Model file for the job. Use its own axes, mm. Face numbers are marked on the shaded views. Round coordinates to 2 decimals unless told otherwise and drop trailing zeros. Write each loop counter-clockwise with the first axis right and the second up, starting at its lowest first coordinate (ties: lowest second). Pieces come first, ordered by that corner, then holes.
```python
from build123d import *

# Parameters (mm, degrees)
F0_R     = 53.4294983316
F0_R_2   = 51.6
F1_DEPTH = 3
F3_R     = 53.9566734819
F4_DEPTH = 2
F5_R     = 1.99999
F6_R     = 37.4035262833
F7_DEPTH = 3
F8_SIZE2 = 1
F8_SIZE  = 1


# Not quite as in the source:
# - a fillet or chamfer is up to 0.001 mm smaller than in the source, because OpenCascade refuses the exact size


with BuildPart() as f1:
    # F0 (on Top) → F1 (new body)
    with BuildSketch(Plane.XY):
        Circle(F0_R)
        Circle(F0_R_2, mode=Mode.SUBTRACT)
    extrude(amount=-F1_DEPTH)

    # F3 (on offset) → F4 (join)
    with BuildSketch(Plane.XY):
        Circle(F3_R)
    extrude(amount=F4_DEPTH)

    # F5 (radius 2 in the source; OpenCascade refuses exactly that, so slightly less here)
    f5_edges = [f1.edges().sort_by_distance(p)[0] for p in [
        (-53.956673, 0, 2),
    ]]
    fillet(f5_edges, radius=F5_R)

    # F6 (on offset) → F7 (cut)
    with BuildSketch(Plane.XY):
        Circle(F6_R)
    extrude(amount=F7_DEPTH, mode=Mode.SUBTRACT)

    # F8
    f8_edges = [f1.edges().sort_by_distance(p)[0] for p in [
        (-37.403526, 0, 2),
    ]]
    chamfer(f8_edges, length=F8_SIZE, length2=F8_SIZE2)


solid = f1.part
```
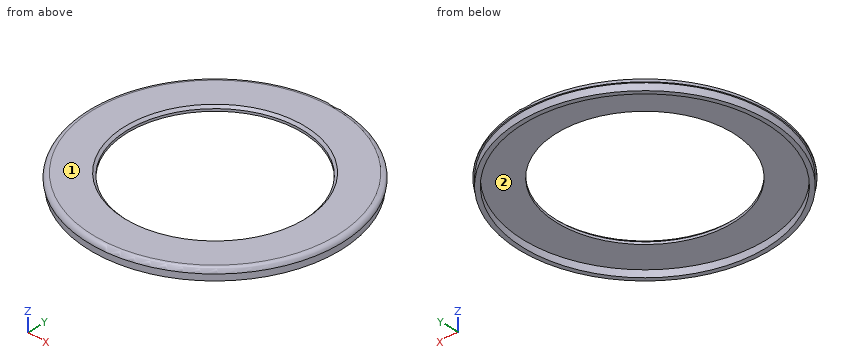
1) Wall check: probe 1 along Y at (x, z) = (0, -1.2); probe 2 along Y at (x, z) = (0, 0.3); probe 3 along Z at (x, y) = (14, -49). Give the ranges that are in metal, low to high.
2) Cut at C-C on z = -1.8. List the corners of the cut face in (x, y).
3) Pull direction Y, two halves, no side cores. Call the marked faces 1 and 2: released by +Y, released by -Y, zero draft, split by the parting line, or undercut.
4) Flat gauge pins, fed straight in: pin 1 Ø2 at (x, z) = (22, -1.5) entering from +Y; pin 2 Ø3 at (y, z) = (-39.5, -1) entering from +X; pin 3 Ø1 at (x, z) = (-13, -2.5) entering from +Y. Where does each tip first touch, or does it go through?
Result sheet:
1. probe 1: y = -53.43 to -51.6, 51.6 to 53.43
1. probe 2: y = -53.93 to -37.4, 37.4 to 53.93
1. probe 3: z = 0 to 2
2. outline: circle Ø106.86 at (0, 0); hole circle Ø103.2 at (0, 0)
3. face 1: zero draft
3. face 2: undercut
4. pin 1: stops at y = 49.13
4. pin 2: stops at x = 37.92
4. pin 3: stops at y = 51.95
